Geometry check sheet. Reference: the model listing, model coordinates, mm. Face numbers are marked on the shaded views. A direction names the side the tool comes from. Give positions to 0.01 mm unless a question says otherwise; leave off trailing zeros. Order: outer loops, then holes, each group sorted by start corner. A loop starts at its lowest first (then second) coordinate and runs counter-clockwise, first axis right, second up.
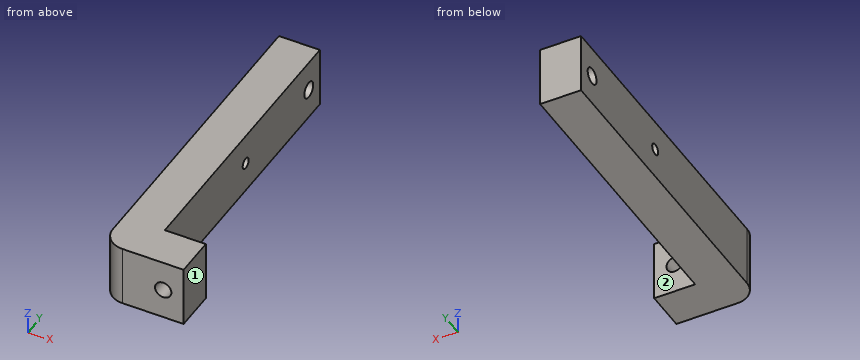
from build123d import *

# Parameters (mm, degrees)
BOSS_EXTRUDE1_DEPTH = 15
FILLET1_R           = 5
SKETCH2_W           = 10
SKETCH2_H           = 15
BOSS_EXTRUDE2_DEPTH = 40
SKETCH3_R           = 2
CUT_EXTRUDE1_DEPTH  = 81
SKETCH4_R           = 2
CUT_EXTRUDE2_DEPTH  = 21
SKETCH5_R           = 1.35
CUT_EXTRUDE3_DEPTH  = 21


with BuildPart() as part:
    # Sketch1 → Boss-Extrude1 (new body)
    with BuildSketch(Plane.XY):
        Polygon((0, 20), (0, -10), (10, -10), (10, -20), (-10, -20), (-10, 20), align=None)
    extrude(amount=BOSS_EXTRUDE1_DEPTH)

    # Fillet1
    fillet1_edges = [part.edges().sort_by_distance(p)[0] for p in [
        (-10, -20, 7.5),
    ]]
    fillet(fillet1_edges, radius=FILLET1_R)

    # Sketch2 → Boss-Extrude2 (add)
    with BuildSketch(Plane(origin=(0, 20, 0), x_dir=(1, 0, 0), z_dir=(0, 1, 0))):
        with Locations((-5, -7.5)):
            Rectangle(SKETCH2_W, SKETCH2_H)
    extrude(amount=BOSS_EXTRUDE2_DEPTH)

    # Sketch3 → Cut-Extrude1 (cut, through all)
    with BuildSketch(Plane.XZ.offset(20)):
        with Locations((5, 7.5)):
            Circle(SKETCH3_R)
    extrude(amount=-CUT_EXTRUDE1_DEPTH, mode=Mode.SUBTRACT)

    # Sketch4 → Cut-Extrude2 (cut, through all)
    with BuildSketch(Plane.ZY.offset(10)):
        with Locations((7.5, 55)):
            Circle(SKETCH4_R)
    extrude(amount=-CUT_EXTRUDE2_DEPTH, mode=Mode.SUBTRACT)

    # Sketch5 → Cut-Extrude3 (cut, through all)
    with BuildSketch(Plane.ZY.offset(10)):
        with Locations((7.5, 26.5)):
            Circle(SKETCH5_R)
    extrude(amount=-CUT_EXTRUDE3_DEPTH, mode=Mode.SUBTRACT)


solid = part.part
Item 1: Set-up check for the marked faces 1 and 2: record each of +Z, -Z, +X, -X, +Y, -Y from which the full face is reachable in a straight line by a thin tool's end or side.
Reported:
face 1: +Z, -Z, +X, +Y, -Y
face 2: +Z, -Z, +X, +Y
Item 2: Sectioned sample at A-A (z = 7.5). Enter the section's corners in (x, y).
Reported:
outline: (-10, -15) arc R5 ccw to (-5, -20) - (3, -20) - (3, -10) - (0, -10) - (0, 25.15) - (-10, 25.15) - close; (-10, 27.85) - (0, 27.85) - (0, 53) - (-10, 53) - close; (-10, 57) - (0, 57) - (0, 60) - (-10, 60) - close; (7, -20) - (10, -20) - (10, -10) - (7, -10) - close
Item 3: Scan lines: L1, parallel to Y at x = -3.25, z = 7.5; L2, parallel to Y at x = -7, z = 7.5; L3, parallel to X at y = 26.5, z = 9. Record each from-to range of solid material in increasing order.
Reported:
L1: y = -20 to 25.15, 27.85 to 53, 57 to 60
L2: y = -19.58 to 25.15, 27.85 to 53, 57 to 60
L3: x = -10 to 0
Item 4: Sectioned sample at D-D (x = -1). Enter the section's corners in (y, z), and give its area (3 significant figures).
Reported:
outline: (-20, 0) - (60, 0) - (60, 15) - (-20, 15) - close; hole circle Ø2.7 at (26.5, 7.5); hole circle Ø4 at (55, 7.5)
area: 1,180 mm2
Item 5: Sectioned sample at C-C (y = 55). Enter the section's corners in (x, z).
Reported:
outline: (-10, 0) - (0, 0) - (0, 5.5) - (-10, 5.5) - close; (-10, 9.5) - (0, 9.5) - (0, 15) - (-10, 15) - close
Item 6: Gauge pin test, flat ends, axial feed: pin 1 (5 mm diameter, centred on y = 30, z = 12.5, fed in from +X); pin 2 (2 mm diameter, centred on y = 26.5, z = 7.5, fed in from -X); pin 3 (5 mm diameter, centred on x = 6, z = 9, fed in from +Y). Record the tip position at first contact, or that the pin passes through.
Reported:
pin 1: stops at x = 0
pin 2: passes through
pin 3: stops at y = -10
Item 7: Sectioned sample at B-B (x = 5). Enter the section's corners in (y, z), and give its area (3 significant figures).
Reported:
outline: (-20, 0) - (-10, 0) - (-10, 5.5) - (-20, 5.5) - close; (-20, 9.5) - (-10, 9.5) - (-10, 15) - (-20, 15) - close
area: 110 mm2
